Work out the finished part from the listing and answer in its coordinate system (mm). Face numbers are marked on the shaded views. A direction names the side the tool comes from. Coordinates: 2 decimals unless noted, no trailing zeros. Order: outer loops, then holes, each group sorted by start corner. A loop starts at its lowest first (then second) coordinate and runs counter-clockwise, first axis right, second up.
1. The part is cut by section C-C, the plane y = 0. Give the vertices of the cut face in (x, z).
2. Determine the mould class of the marked faces 1, 2 and 3 for opening direction X: +X half, -X half, draft (parallel to the pull), parting line (faces both ways), or undercut.
3. A tool of negligible diameter and unlimited length cuts with its end or side. For the marked faces 4, 5, 6 and 7, from which of +Z, -Z, +X, -X, +Y, -Y can it reach the whole face along a straight path? Write none if from no direction.
4. Find the intervals of material crossed by probe 1 along X at (y, z) = (11, 7.5); probe 2 along Y at (x, z) = (-33.5, 3.25); probe 3 along X at (y, z) = (-0.5, 16.5), in increasing order.
5. Flat-ended cylindrical pins translate along their axes: pin 1 Ø5 at (y, z) = (-7.5, 20.5) entering from +X; pin 2 Ø23 at (x, y) = (-38, 12.5) entering from +Z; pin 3 Ø8 at (x, y) = (42.5, -17) entering from +Z; pin 4 Ø9 at (x, y) = (-33.55, 15.45) entering from -Z. Find the tip coordinate at first contact, or state that the pin passes through.
6. The part is cut by section D-D, the plane z = 19.5. Give the vertices of the cut face in (x, y), then the cut area to 3 significant figures.
7. The part is cut by section B-B, the plane z = 4. Give the vertices of the cut face in (x, y), then the cut area to 3 significant figures.
8. The part is cut by section A-A, the plane x = 14. Give the vertices of the cut face in (y, z), then the cut area to 3 significant figures.
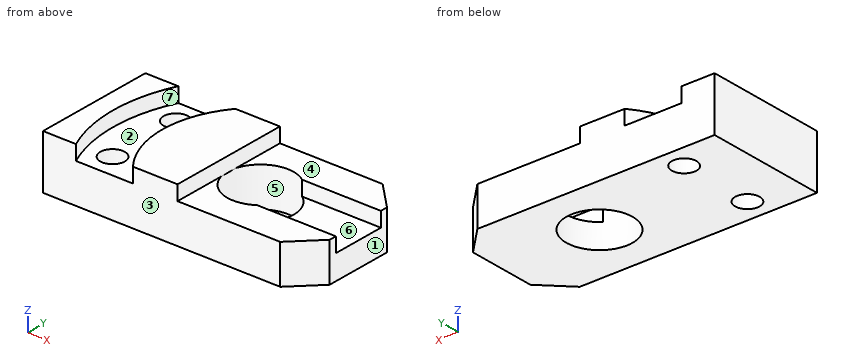
```python
from build123d import *

# Parameters (mm, degrees)
SKETCH1_W           = 108
SKETCH1_H           = 50
BOSS_EXTRUDE1_DEPTH = 22
SKETCH2_W           = 53
SKETCH2_H           = 50
CUT_EXTRUDE1_DEPTH  = 6
CUT_EXTRUDE2_REACH  = 63.62
SKETCH3_R           = 13.5
SKETCH4_W           = 40
SKETCH4_H           = 22
CUT_EXTRUDE3_DEPTH  = 6
CHAMFER1_SIZE       = 11
CUT_EXTRUDE4_REACH  = 63.62
SKETCH5_R           = 5


with BuildPart() as part:
    # Sketch1 → Boss-Extrude1 (new body)
    with BuildSketch(Plane.XY):
        Rectangle(SKETCH1_W, SKETCH1_H)
    extrude(amount=BOSS_EXTRUDE1_DEPTH)

    # Sketch2 → Cut-Extrude1 (cut)
    with BuildSketch(Plane.XY.offset(22)):
        with Locations((27.5, 0)):
            Rectangle(SKETCH2_W, SKETCH2_H)
        with BuildLine():
            Line((-17.224989992, 25), (-40.543560573, 25))
            ThreePointArc((-40.543560573, 25), (-46, 0), (-40.543560573, -25))
            Line((-40.543560573, -25), (-17.224989992, -25))
            ThreePointArc((-17.224989992, -25), (-26, 0), (-17.224989992, 25))
        make_face()
    extrude(amount=-CUT_EXTRUDE1_DEPTH, mode=Mode.SUBTRACT)

    # Sketch3 → Cut-Extrude2 (cut, up to next)
    with BuildSketch(Plane.XY.offset(16), mode=Mode.PRIVATE) as cut_extrude2_sk1:
        with Locations((14, 0)):
            Circle(SKETCH3_R)
    cut_extrude2_tool1 = extrude(cut_extrude2_sk1.sketch, amount=-CUT_EXTRUDE2_REACH, mode=Mode.PRIVATE) & part.part
    add(cut_extrude2_tool1.solids().sort_by_distance((14, 0, 16))[0], mode=Mode.SUBTRACT)

    # Sketch4 → Cut-Extrude3 (cut)
    with BuildSketch(Plane.XY.offset(16)):
        with Locations((34, 0)):
            Rectangle(SKETCH4_W, SKETCH4_H)
    extrude(amount=-CUT_EXTRUDE3_DEPTH, mode=Mode.SUBTRACT)

    # Chamfer1
    chamfer1_edges = [part.edges().sort_by_distance(p)[0] for p in [
        (54, -25, 8),
        (54, 25, 8),
    ]]
    chamfer(chamfer1_edges, length=CHAMFER1_SIZE)

    # Sketch5 → Cut-Extrude4 (cut, up to next)
    with BuildSketch(Plane.XY.offset(16), mode=Mode.PRIVATE) as cut_extrude4_sk1:
        with Locations((-33.553101897, 15.45)):
            Circle(SKETCH5_R)
    cut_extrude4_tool1 = extrude(cut_extrude4_sk1.sketch, amount=-CUT_EXTRUDE4_REACH, mode=Mode.PRIVATE) & part.part
    # Sketch5 → Cut-Extrude4 (cut, up to next)
    with BuildSketch(Plane.XY.offset(16), mode=Mode.PRIVATE) as cut_extrude4_sk2:
        with Locations((-33.553101897, -15.45)):
            Circle(SKETCH5_R)
    cut_extrude4_tool2 = extrude(cut_extrude4_sk2.sketch, amount=-CUT_EXTRUDE4_REACH, mode=Mode.PRIVATE) & part.part
    add(cut_extrude4_tool1.solids().sort_by_distance((-33.553102, 15.45, 16))[0], mode=Mode.SUBTRACT)
    add(cut_extrude4_tool2.solids().sort_by_distance((-33.553102, -15.45, 16))[0], mode=Mode.SUBTRACT)


solid = part.part
```
Geometry says:
1. outline: (-54, 0) - (0.5, 0) - (0.5, 16) - (1, 16) - (1, 22) - (-26, 22) - (-26, 16) - (-46, 16) - (-46, 22) - (-54, 22) - close; (27.5, 0) - (54, 0) - (54, 10) - (27.5, 10) - close
2. face 1: +X half
2. face 2: undercut
2. face 3: draft
3. face 4: +Z, +X, +Y, -Y
3. face 5: -Z
3. face 6: +Z, +X
3. face 7: +Z
4. probe 1: x = -54 to -35.83, -31.27 to 6.17, 21.83 to 54
4. probe 2: y = -25 to -20.45, -10.45 to 10.45, 20.45 to 25
4. probe 3: x = -54 to -46, -26 to 1
5. pin 1: stops at x = 1
5. pin 2: stops at z = 22
5. pin 3: stops at z = 16
5. pin 4: passes through
6. outline: (-54, -25) - (-40.54, -25) arc R60 cw to (-40.54, 25) - (-54, 25) - close; (-17.22, -25) - (1, -25) - (1, 25) - (-17.22, 25) arc R40 ccw to start
6. area: 1,700 mm2
7. outline: (-54, -25) - (43, -25) - (54, -14) - (54, 14) - (43, 25) - (-54, 25) - close; hole circle Ø10 at (-33.55, -15.45); hole circle Ø10 at (-33.55, 15.45); hole circle Ø27 at (14, 0)
7. area: 4,550 mm2
8. outline: (-25, 0) - (-13.5, 0) - (-13.5, 16) - (-25, 16) - close; (13.5, 0) - (25, 0) - (25, 16) - (13.5, 16) - close
8. area: 368 mm2
